Geometry: final body of the model. Coordinates: model frame, mm. A direction names the side the tool comes from. Round coordinates to 2 decimals unless told otherwise and drop trailing zeros. Loops run counter-clockwise (first coordinate to the right, second up) from the corner with the lowest first, then second, coordinate; pieces in that order, holes last. Notation, with made-up numbers: M 72.5,19 L 99.5,19 A17 ccw 99.5,33 Z; hole C 14.25,-26.5 d2. An arc over 180 degrees is marked long. Answer as a JSON object with one key per item and string values.
Autodesk Inventor part; units mm, degrees
ref_plane "YZ Plane" through (0, 0, 0) normal (1, 0, 0) x (0, 1, 0)
ref_plane "XZ Plane" through (0, 0, 0) normal (0, 1, 0) x (-1, 0, 0)
ref_plane "XY Plane" through (0, 0, 0) normal (0, 0, 1) x (1, 0, 0)
sketch "Sketch1" plane through (0, 0, 0) normal (0, 1, 0) x (-1, 0, 0)
  circle A0 centre (0, 0) radius 1.5
  line L0 (0, 3.1754) -> (2.75, 1.5877)
  line L1 (2.75, 1.5877) -> (2.75, -1.5877)
  line L2 (2.75, -1.5877) -> (0, -3.1754)
  line L3 (0, -3.1754) -> (-2.75, -1.5877)
  line L4 (-2.75, -1.5877) -> (-2.75, 1.5877)
  line L5 (-2.75, 1.5877) -> (0, 3.1754)
  dimension "d0" = 3
  dimension "d4" = 5.5
extrude "Extrusion1" add sketch "Sketch1" along normal blind 25
thread "Thread2"
sketch "Sketch3" plane through (0, 0, 0) normal (0, -1, 0) x (1, 0, 0)
  circle A0 centre (0, 0) radius 1.5066
extrude "Extrusion3" add sketch "Sketch3" along normal blind 6
thread "Thread3"
chamfer "Chamfer1" distance 0.3 angle 45 1 edges at (-1.5066, -6, 0)
properties part number "Spacer" material "Nylon 6"
1) First-contact query: pin 1 (0.9 mm diameter, centred on x = -0.5, z = -0.5, fed in from +Y); pin 2 (3 mm diameter, centred on x = -2, y = 21.5, fed in from -Z). Flat tips, straight axial feed; report the tip coordinate or a pass-through.
Geometry results:
{"pin 1": "y = 0", "pin 2": "z = -2.89"}
2) Pull-direction query (X, two-part tool) for faces 4 (the face through (1.3, 25, -1.4)), 5 (the face through (0, 0, 0)), 6 (the face through (1.394, 12.325, 2.37)); classes: +X half, -X half, draft (parallel to the pull), parting line (faces both ways), or undercut.
Geometry results:
{"face 4": "draft", "face 5": "undercut", "face 6": "+X half"}
3) Line query: probe 1 along Y at (x, z) = (-2.25, -1); probe 2 along Y at (x, z) = (0, -1); probe 3 along Z at (x, y) = (-0.15, 13.5). Output: solid intervals per line, ascending.
Geometry results:
{"probe 1": "0 to 25", "probe 2": "-6 to 0", "probe 3": "-3.09 to -1.49, 1.49 to 3.09"}
4) Cut plane D-D on z = 2.25. Return the cut outline in (x, y).
Geometry results:
{"outline": "M -1.6,0 L 1.6,0 L 1.6,25 L -1.6,25 Z"}
5) Cut plane B-B on z = 0. Return the cut outline in (x, y).
Geometry results:
{"outline": "M -2.75,0 L -1.51,0 L -1.51,-5.7 L -1.21,-6 L 1.21,-6 L 1.51,-5.7 L 1.51,0 L 2.75,0 L 2.75,25 L 1.5,25 L 1.5,0 L -1.5,0 L -1.5,25 L -2.75,25 Z"}
6) Cut plane A-A on y = 8. Return the cut outline in (x, z).
Geometry results:
{"outline": "M -2.75,-1.59 L 0,-3.18 L 2.75,-1.59 L 2.75,1.59 L 0,3.18 L -2.75,1.59 Z; hole C 0,0 d3"}
7) Set-up query: faces 1 (the face through (1.3, 0, -1.4)), 2 (the face through (1.5, 12.32, -0.07)), 3 (the face through (1.36, 12.32, -2.39)). Return all of +Z, -Z, +X, -X, +Y, -Y with unobstructed straight access to the full face (end or side cutting, diameter ignored); none if empty.
Geometry results:
{"face 1": "-Y", "face 2": "+Y", "face 3": "-Z, +X, +Y, -Y"}
8) Cut plane C-C on y = -2. Return the cut outline in (x, z), and give its area (3 significant figures).
Geometry results:
{"outline": "C 0,0 d3.01", "area": "7.13 mm2"}
